The listing builds one solid part. Answer for the finished solid, in the listing's coordinates (mm). A direction names the side the tool comes from. Give positions to 0.01 mm unless a question says otherwise; leave off trailing zeros. Order: outer loops, then holes, each group sorted by start corner. A loop starts at its lowest first (then second) coordinate and runs counter-clockwise, first axis right, second up. Notation, with made-up numbers: (86.5, 24) - (131.5, 24) arc R3 cw to (131.5, 28) - close; hole circle Ø6 at (18, 68). An arc over 180 degrees is marked (long way). Answer as a JSON object with one key per item and string values. Group by question number.
Q1. A cutting plane is placed at A-A, the plane z = 3.6. Give the vertices of the cut face in (x, y).
Q2. Given pin 1 (3 mm diameter, centred on x = 0, y = 0, fed in from +Z); pin 2 (1.6 mm diameter, centred on y = -8, z = 0.5, fed in from +X); pin 3 (1.5 mm diameter, centred on x = 1, y = -3.5, fed in from -Z); pin 4 (1 mm diameter, centred on x = 15, z = 4, fed in from -Y), each flat-ended and moving along its own axis, determine where each tip first touches the part or whether it passes through.
Q3. The mould has two halves that part along X. Classify faces 1 (the face through (15, 4.166, 4)), 2 (the face through (-5, -7, 1)), 3 (the face through (3.767, -12, 2)): released by +X, released by -X, zero draft, split by the parting line, or undercut.
Q4. A cutting plane is placed at D-D, the plane z = 0.75. Give the vertices of the cut face in (x, y).
Q5. Consider line 1 (X direction, y = 3.5, z = 2.45); line 2 (Z direction, x = 14.5, y = 3); line 3 (X direction, y = -8.5, z = 1.25). Determine where each line is inside the solid, lowest interval first.
Q6. For faces 4 (the face through (10, 1.569, 2)), 5 (the face through (3, -4, 1)), 6 (the face through (0, -2, 1)), 7 (the face through (11, 1, 3)), 8 (the face through (-3, 4, 1)), determine the directions among +Z, -Z, +X, -X, +Y, -Y from which every point of the face is accessible in a straight line to the end or side of a thin tool.
Q7. A cutting plane is placed at B-B, the plane x = 1.75. Give the vertices of the cut face in (y, z), and give its area (3 significant figures).
from build123d import *

# Parameters (mm, degrees)
SKETCH_1_R      = 5
SKETCH_1_R_2    = 2
EXTRUDE_1_DEPTH = 1.5
SKETCH_1_3_W    = 0.979922275
SKETCH_1_3_H    = 1.483986981
EXTRUDE_2_DEPTH = 3
EXTRUDE_3_DEPTH = 5


with BuildPart() as part:
    # Sketch 1 → Extrude 1 (new body)
    # profile 1 of 3: a face of its own
    with BuildSketch(Plane.XY):
        Circle(SKETCH_1_R)
        Circle(SKETCH_1_R_2, mode=Mode.SUBTRACT)
    # profile 2 of 3: a face of its own
    with BuildSketch(Plane.XY):
        with BuildLine():
            ThreePointArc((0, -5), (-1.902759219, -4.623797936), (-3.51918966, -3.551802942))
            Line((-3.51918966, -3.551802942), (-3.51918966, -12.678202106))
            Line((-3.51918966, -12.678202106), (3.767394394, -12.678202106))
            Line((3.767394394, -12.678202106), (3.767394394, -11.194215125))
            Line((3.767394394, -11.194215125), (0, -11.194215125))
            Line((0, -11.194215125), (0, -5))
        make_face()
    # profile 3 of 3: a face of its own
    with BuildSketch(Plane.XY):
        with BuildLine():
            Line((4.103232797, 5), (0, 5))
            ThreePointArc((0, 5), (2.928570542, 4.052588627), (4.747316669, 1.569389833))
            Line((4.747316669, 1.569389833), (14.616295983, 1.569389833))
            Line((14.616295983, 1.569389833), (14.616295983, 3.323351723))
            Line((14.616295983, 3.323351723), (11.529062921, 3.323351723))
            Line((11.529062921, 3.323351723), (11.529062921, 4.354010329))
            Line((11.529062921, 4.354010329), (4.103232797, 5))
        make_face()
    extrude(amount=EXTRUDE_1_DEPTH)

    # Sketch 1_3 → Extrude 2 (add)
    with BuildSketch(Plane.XY):
        with BuildLine():
            ThreePointArc((-3.51918966, -3.551802942), (-4.614972822, -1.924064929), (-5, 0))
            Line((-5, 0), (-5, -12.678202106))
            Line((-5, -12.678202106), (-3.51918966, -12.678202106))
            Line((-3.51918966, -12.678202106), (-3.51918966, -3.551802942))
        make_face()
        with BuildLine():
            Line((14.616295983, 1.569389833), (4.747316669, 1.569389833))
            ThreePointArc((4.747316669, 1.569389833), (4.880000714, 1.088849406), (4.964172837, 0.597484763))
            Line((4.964172837, 0.597484763), (15.542189383, 0.597484763))
            Line((15.542189383, 0.597484763), (15.542189383, 4.165774783))
            Line((15.542189383, 4.165774783), (14.616295983, 4.165774783))
            Line((14.616295983, 4.165774783), (14.616295983, 3.323351723))
            Line((14.616295983, 3.323351723), (14.616295983, 1.569389833))
        make_face()
        with Locations((4.257355532, -11.936208616)):
            Rectangle(SKETCH_1_3_W, SKETCH_1_3_H)
    extrude(amount=EXTRUDE_2_DEPTH)

    # Sketch 1_4 → Extrude 3 (add)
    with BuildSketch(Plane.XY):
        Polygon((-3.51918966, -12.678202106), (-5, -12.678202106), (-5, -14.27668016), (5.501186974, -14.27668016), (5.501186974, -11.194215125), (4.747316669, -11.194215125), (4.747316669, -12.678202106), (3.767394394, -12.678202106), align=None)
        with BuildLine():
            Line((15.542189383, 0.597484763), (4.964172837, 0.597484763))
            ThreePointArc((4.964172837, 0.597484763), (4.991035173, 0.299278978), (5, 0))
            Line((5, 0), (16.481935348, 0))
            Line((16.481935348, 0), (16.481935348, 5.008197844))
            Line((16.481935348, 5.008197844), (14.616295983, 5.008197844))
            Line((14.616295983, 5.008197844), (14.616295983, 4.165774783))
            Line((14.616295983, 4.165774783), (15.542189383, 4.165774783))
            Line((15.542189383, 4.165774783), (15.542189383, 0.597484763))
        make_face()
    extrude(amount=EXTRUDE_3_DEPTH)


solid = part.part
Reply:
{
 "1": {"outline": "(-5, -14.28) - (5.5, -14.28) - (5.5, -11.19) - (4.75, -11.19) - (4.75, -12.68) - (-5, -12.68) - close; (4.96, 0.6) arc R5 cw to (5, 0) - (16.48, 0) - (16.48, 5.01) - (14.62, 5.01) - (14.62, 4.17) - (15.54, 4.17) - (15.54, 0.6) - close"},
 "2": {"pin 1": "passes through", "pin 2": "stops at x = 0", "pin 3": "stops at z = 0", "pin 4": "stops at y = 0"},
 "3": {"face 1": "zero draft", "face 2": "released by -X", "face 3": "undercut"},
 "4": {"outline": "(-5, -14.28) - (5.5, -14.28) - (5.5, -11.19) - (0, -11.19) - (0, -5) arc R5 ccw to (5, 0) - (16.48, 0) - (16.48, 5.01) - (14.62, 5.01) - (14.62, 3.32) - (11.53, 3.32) - (11.53, 4.35) - (4.1, 5) - (0, 5) arc R5 ccw to (-5, 0) - close; hole circle Ø4 at (0, 0)"},
 "5": {"line 1": "x = 14.62 to 16.48", "line 2": "z = 0 to 1.5", "line 3": "x = -5 to 0"},
 "6": {"face 4": "+Z, -X, +Y", "face 5": "+Z, -Z, +X", "face 6": "+Z, -Z", "face 7": "+Z, -X", "face 8": "+Z, -Z, -X, +Y"},
 "7": {"outline": "(-14.28, 0) - (-11.19, 0) - (-11.19, 1.5) - (-12.68, 1.5) - (-12.68, 5) - (-14.28, 5) - close; (-4.68, 0) - (-0.97, 0) - (-0.97, 1.5) - (-4.68, 1.5) - close; (0.97, 0) - (5, 0) - (5, 1.5) - (0.97, 1.5) - close", "area": "21.8 mm^2"}
}
